Check sheet for the modelled part. Datum: model origin and axes. Units: mm. Face numbers are marked on the shaded views. Round coordinates to 2 decimals unless told otherwise and drop trailing zeros. Loops run counter-clockwise (first coordinate to the right, second up) from the corner with the lowest first, then second, coordinate; pieces in that order, holes last. Notation, with made-up numbers: (65, 75.5) - (117, 75.5) arc R17 ccw to (117, 87.5) - close; hole circle Ø8 at (-15, -29). An arc over 180 degrees is marked (long way). Put each result on its own line as item: value. Start each with the question number.
Item 1: Draft check along Z on the marked faces 1 and 2. Enter one of: pulls with the +Z half, pulls with the -Z half, needs draft (parallel to the pull), parting line crosses it, or undercut.
Item 2: Section check B-B, the plane z = 0. Record the cut outline in (x, y).
Item 3: Gauge pin test, flat ends, axial feed: pin 1 Ø2 at (x, y) = (2.5, 10.5) entering from -Z; pin 2 Ø1 at (y, z) = (0.5, 2.5) entering from +X; pin 3 Ø2 at (y, z) = (-7, 2) entering from -X. Record the tip position at first contact, or that the pin passes through.
Item 4: Material ranges on line 1 along Z through (x, y) = (0, -2.5); line 2 along Z through (x, y) = (-1.75, -22.5); line 3 along X through (y, z) = (21, 2.75), recorded low to high.
Item 5: Section check C-C, the plane y = 2. Record the cut outline in (x, z), and give its area (3 significant figures).
Item 6: Section check A-A, the plane x = 0. Record the cut outline in (y, z), and give its area (3 significant figures).
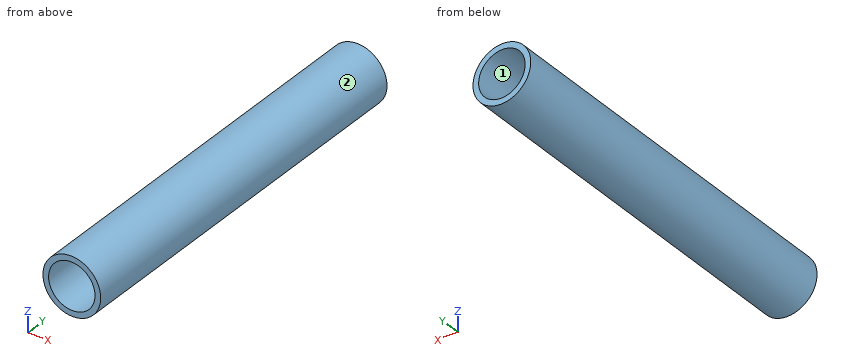
from build123d import *

# Parameters (mm, degrees)
F0_R     = 3.81
F1_DEPTH = 25.4
F3_DEPTH = 25.4
F4_R     = 3.0643911348
F5_DEPTH = 50.801


# Not quite as in the source:
# - the program builds the solid bodies; features that only make, move or delete a surface that nothing else refers to are left out


with BuildPart() as f1:
    # F0 (on Front) → F1 (new body)
    with BuildSketch(Plane.XZ):
        Circle(F0_R)
    extrude(amount=F1_DEPTH)

    # F3 (add): a face of the model
    f3_faces = [f1.faces().sort_by_distance(p)[0] for p in [
        (0, 0, 0),
    ]]
    extrude(f3_faces, amount=F3_DEPTH)

    # F4 (on face) → F5 (cut, through all)
    with BuildSketch(Plane(origin=(0, 25.4, 0), x_dir=(-1, 0, 0), z_dir=(0, 1, 0))):
        Circle(F4_R)
    extrude(amount=-F5_DEPTH, mode=Mode.SUBTRACT)


solid = f1.part
Check result:
1. face 1: undercut
1. face 2: parting line crosses it
2. outline: (-3.81, -25.4) - (-3.06, -25.4) - (-3.06, 25.4) - (-3.81, 25.4) - close; (3.06, -25.4) - (3.81, -25.4) - (3.81, 25.4) - (3.06, 25.4) - close
3. pin 1: z = -3.5
3. pin 2: x = 3.24
3. pin 3: x = -3.68
4. line 1: -3.81 to -3.06, 3.06 to 3.81
4. line 2: -3.38 to -2.52, 2.52 to 3.38
4. line 3: -2.64 to -1.35, 1.35 to 2.64
5. outline: circle Ø7.62 at (0, 0); hole circle Ø6.13 at (0, 0)
5. area: 16.1 mm²
6. outline: (-25.4, -3.81) - (25.4, -3.81) - (25.4, -3.06) - (-25.4, -3.06) - close; (-25.4, 3.06) - (25.4, 3.06) - (25.4, 3.81) - (-25.4, 3.81) - close
6. area: 75.8 mm²
